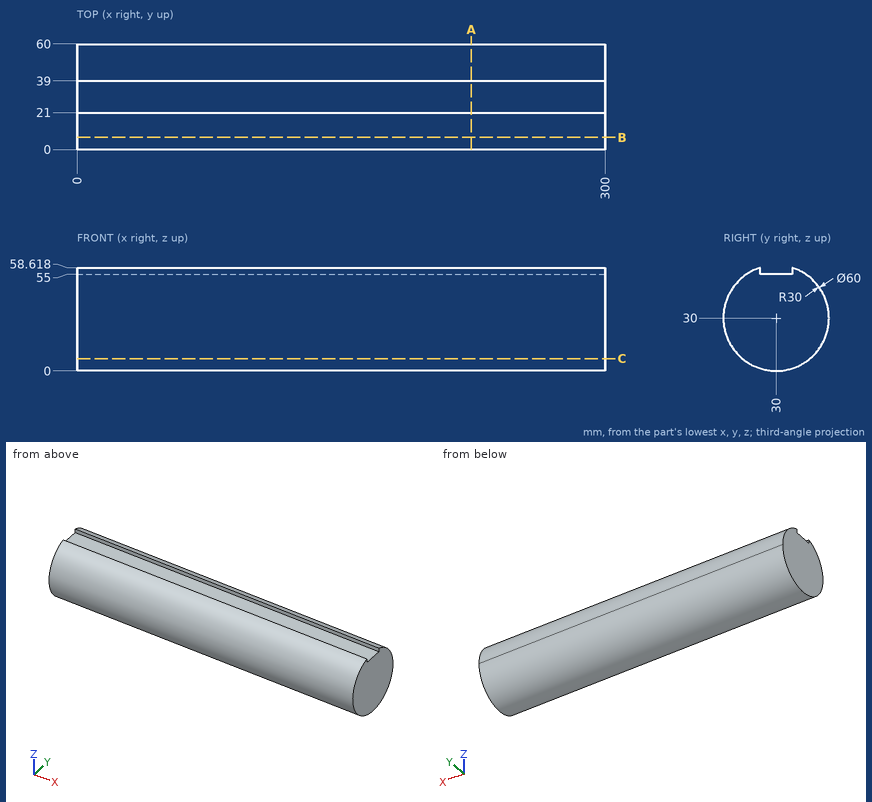
Design review of the part shown in the three views and the two pictorial views. Dimensions are in mm from the part's minimum x, y and z. Give positions to 0.01 mm unless a question says otherwise; leave off trailing zeros. Loops run counter-clockwise (first coordinate to the right, second up) from the corner with the lowest first, then second, coordinate; pieces in that order, holes last. Notation, with made-up numbers: M -31.5,27.5 L 26.5,27.5 A16 ccw 26.5,51.5 Z; hole C 36.25,48 d9. An arc over 180 degrees is marked long. Write item = value, one per line.
Q1. We need section A-A (x = 224). Give the boundary of the cut face in (y, z).
Output values:
outline = M 21,55 L 21,58.62 A30 ccw long 60,30 A30 ccw 39,58.62 L 39,55 Z
Q2. We need section B-B (y = 7). Give the boundary of the cut face in (x, z).
Output values:
outline = M 0,10.74 L 300,10.74 L 300,49.26 L 0,49.26 Z
Q3. Insertion check: pin 1 (3 mm diameter, centred on x = 202, y = 14, fed in from -Z); pin 2 (3 mm diameter, centred on x = 204, y = 40.5, fed in from -Z); pin 3 (1.8 mm diameter, centred on x = 130.5, z = 57.5, fed in from +Y); pin 4 (3 mm diameter, centred on y = 19, z = 47.5, fed in from -X). Each pin has a flat end and moves straight along its axis. Give the tip position at first contact, or say it passes through.
Output values:
pin_1 = 3.74
pin_2 = 1.38
pin_3 = 43.87
pin_4 = 0
Q4. To check wall thickness, follow line 1 (Y direction, x = 198.5, z = 17); line 2 (Z direction, x = 248, y = 34); line 3 (Z direction, x = 240, y = 4.5). State the ranges of each line that lie inside material, in increasing order. Write a range as [from, to].
Output values:
line_1 = [2.96, 57.04]
line_2 = [0.27, 55]
line_3 = [14.2, 45.8]
